Source: CAD feature listing. Evaluate the final solid. Frame: model axes, mm. Face numbers are marked on the shaded views. Coordinates: 2 decimals unless noted, no trailing zeros. Order: outer loops, then holes, each group sorted by start corner. A loop starts at its lowest first (then second) coordinate and runs counter-clockwise, first axis right, second up. Notation, with made-up numbers: (48.25, 1.5) - (63.25, 1.5) arc R20 cw to (63.25, 10.5) - close; hole circle Ø2 at (16.25, 76.5). An arc over 180 degrees is marked (long way). One line per question, with ' | ' between items. Start each with the question number.
(1) Section C-C (x = -63). Return the cut outline in (y, z).
(2) Draft query along X for the marked faces 1, 2 and 3. Return one class per face: +X half, -X half, draft (parallel to the pull), parting line (faces both ways), or undercut.
(3) Section D-D (x = -39). Return the cut outline in (y, z).
(4) Section A-A (x = 49). Return the cut outline in (y, z), then the cut area to 3 significant figures.
(5) Line query: line 1 along X through (y, z) = (16, 23.5); line 2 along X through (y, z) = (7.5, 27.5); line 3 along Z through (x, y) = (-20.5, 11.5). Output: solid intervals per line, ascending.
(6) Contact query for flat-ended pins moving along their axis: P1, Ø5.5, axis at x = 12.5, y = 6.5, coming from the -Z side; P2, Ø0.8, axis at x = 35.5, y = 18.5, coming from the +Z side; P3, Ø12, axis at x = 47, z = 27, coming from the +Y side; P4, Ø5, axis at x = -29, z = 37.5, coming from the +Y side. Output: stop coordinate, or through.
(7) Section B-B (x = -15.5). Return the cut outline in (y, z).
from build123d import *

# Parameters (mm, degrees)
F1_DEPTH      = 76.2
F1_DEPTH_BACK = 76.2
F3_D          = 6.5278
F3_DEPTH      = 15.875
F3_TIP        = 1.9611489744
F5_D          = 6.5278
F5_DEPTH      = 15.875
F5_TIP        = 1.9611489744
F7_DEPTH      = 18.543
F8_R          = 4.3561
F9_DEPTH      = 18.543


with BuildPart() as f1:
    # F0 (on Right) → F1 (new body, two sides)
    with BuildSketch(Plane.YZ) as f1_sk:
        Polygon((0, 38.862), (0, 0), (18.542, 0), (18.542, 32.766), (17.5658409794, 32.766), (16.3086051224, 31.5087641431), (14.8717641431, 32.9456051224), (16.129, 34.2028409794), (16.129, 38.862), align=None)
    extrude(amount=F1_DEPTH)
    extrude(f1_sk.sketch, amount=-F1_DEPTH_BACK)

    # F3
    with Locations(Plane.YZ.offset(76.2)):
        with Locations((8.636, 11.176), (8.636, 26.416)):
            Hole(F3_D / 2, depth=F3_DEPTH)
            with Locations((0, 0, -(F3_DEPTH + F3_TIP / 2))):  # 118° drill point
                Cone(0, F3_D / 2, F3_TIP, mode=Mode.SUBTRACT)

    # F5
    with Locations(Plane(origin=(-76.2, 0, 0), x_dir=(0, -1, 0), z_dir=(-1, 0, 0))):
        with Locations((-8.636, 26.416), (-8.636, 11.176)):
            Hole(F5_D / 2, depth=F5_DEPTH)
            with Locations((0, 0, -(F5_DEPTH + F5_TIP / 2))):  # 118° drill point
                Cone(0, F5_D / 2, F5_TIP, mode=Mode.SUBTRACT)

    # F6 (on face) → F7 (cut, through all)
    with BuildSketch(Plane.XZ):
        Polygon((-34.93135, 0.79375), (-35.7251, 0), (35.7251, 0), (34.93135, 0.79375), align=None)
    extrude(amount=-F7_DEPTH, mode=Mode.SUBTRACT)

    # F8 (on face) → F9 (cut, through all)
    with BuildSketch(Plane(origin=(0, 18.542, 0), x_dir=(-1, 0, 0), z_dir=(0, 1, 0))):
        with Locations((-49.2125, 23.7998)):
            Circle(F8_R)
        with Locations((49.2125, 23.7998)):
            Circle(F8_R)
    extrude(amount=-F9_DEPTH, mode=Mode.SUBTRACT)


solid = f1.part
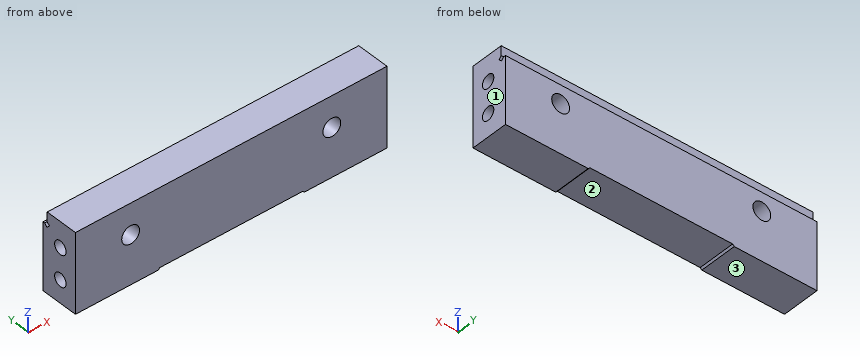
Response values:
1) outline: (0, 0) - (18.54, 0) - (18.54, 32.77) - (17.57, 32.77) - (16.31, 31.51) - (14.87, 32.95) - (16.13, 34.2) - (16.13, 38.86) - (0, 38.86) - close; hole circle Ø6.53 at (8.64, 11.18); hole circle Ø6.53 at (8.64, 26.42)
2) face 1: +X half | face 2: undercut | face 3: draft
3) outline: (0, 0) - (18.54, 0) - (18.54, 32.77) - (17.57, 32.77) - (16.31, 31.51) - (14.87, 32.95) - (16.13, 34.2) - (16.13, 38.86) - (0, 38.86) - close
4) outline: (0, 0) - (18.54, 0) - (18.54, 19.45) - (0, 19.45) - close; (0, 28.15) - (18.54, 28.15) - (18.54, 32.77) - (17.57, 32.77) - (16.31, 31.51) - (14.87, 32.95) - (16.13, 34.2) - (16.13, 38.86) - (0, 38.86) - close | area: 542 mm²
5) line 1: x = -76.2 to -53.56, -44.87 to 44.87, 53.56 to 76.2 | line 2: x = -59.31 to -51.51, -46.91 to 46.91, 51.51 to 59.31 | line 3: z = 0.79 to 38.86
6) P1: stops at z = 0.79 | P2: stops at z = 32.77 | P3: stops at y = 18.54 | P4: stops at y = 16.13
7) outline: (0, 0.79) - (18.54, 0.79) - (18.54, 32.77) - (17.57, 32.77) - (16.31, 31.51) - (14.87, 32.95) - (16.13, 34.2) - (16.13, 38.86) - (0, 38.86) - close
